Autodesk Inventor part; units mm, degrees
ref_plane "YZ Plane" through (0, 0, 0) normal (1, 0, 0) x (0, 1, 0)
ref_plane "XZ Plane" through (0, 0, 0) normal (0, 1, 0) x (-1, 0, 0)
ref_plane "XY Plane" through (0, 0, 0) normal (0, 0, 1) x (1, 0, 0)
ref_plane "Arbeitsebene1" through (-42.5, -18.05, -10) normal (0, -1, 0) x (1, 0, 0)
sketch "Skizze1" plane through (-42.5, -18.05, -10) normal (0, -1, 0) x (1, 0, 0)
  line L0 (45.91, 10.609) -> (59.4818, 10.609) construction
  line L1 (59.4818, 10.609) -> (63.5906, 10.303) construction
  line L2 (63.5906, 10.303) -> (66.1223, 6.4827) construction
  line L3 (66.1223, 6.4827) -> (69.15, 6.4827) construction
  spline S0 degree 4 poles (45.91, 10.609) (59.4818, 10.609) (63.5906, 10.303) (66.1223, 6.4827) (69.15, 6.4827) knots 1 1 1 1 1 2 2 2 2 2
  line L4 (46.0094, 12.5239) -> (59.5812, 12.5239) construction
  line L5 (59.5812, 12.5239) -> (63.69, 12.218) construction
  line L6 (63.69, 12.218) -> (66.2218, 8.3976) construction
  line L7 (66.2218, 8.3976) -> (69.15, 8.1737) construction
  spline S1 degree 4 poles (46.0094, 12.5239) (59.5812, 12.5239) (63.69, 12.218) (66.2218, 8.3976) (69.15, 8.1737) knots 1 1 1 1 1 2 2 2 2 2
  line L8 (46.0094, 12.5239) -> (45.91, 10.609)
  line L9 (69.15, 8.1737) -> (69.15, 6.4827)
  line L10 (42.5, 16.2648) -> (42.5, 4.43)
  point P0 (54.5567, 11.9133)
extrude "Extrusion1" add sketch "Skizze1" along normal mid plane 10
ref_plane "Arbeitsebene2" through (0, 0, 0) normal (0, 0, 1) x (1, 0, 0)
sketch "Skizze2" plane through (0, 0, 0) normal (0, 0, 1) x (1, 0, 0)
  line L0 (12.3, -18.05) -> (-2.05, -18.05)
  circle A0 centre (8.65, -14) radius 1.4
  circle A1 centre (8.65, -18.05) radius 1.6
  point P0 (0, 0)
  dimension "d2" = 3.2
extrude "Extrusion2" cut sketch "Skizze2" along normal mid plane 10 contours A1 L0 | L0 A1
mirror "Spiegeln1" about plane through (26.65, -18.05, -3.5173) normal (1, 0, 0) of "Extrusion1", "Extrusion2"
sketch "Skizze3" plane through (0, 0, 0) normal (0, 0, 1) x (1, 0, 0)
  line L0 (10.2456, -18.1688) -> (7.1543, -18.1688)
  line L1 (7.1543, -18.1688) -> (7.1543, 0.1733)
  line L2 (7.1543, 0.1733) -> (10.2456, 0.1733)
  line L3 (10.2456, 0.1733) -> (10.2456, -18.1688)
  point P0 (0, 0)
  point P1 (7.1543, -17.4817)
extrude "Extrusion3" cut sketch "Skizze3" along normal mid plane 10
fillet "Rundung1" radius 2 2 edges at (10.2456, -13.05, 1.4929) (7.1543, -13.05, 1.5517)
ref_plane "Arbeitsebene3" through (53.3, 0, 0) normal (0, 0, -1) x (-1, 0, 0)
properties part number "60_Planktoscope_Sampleholder_2"
Here's how the part is built. I have some questions about the finished solid (model axes, mm). A direction names the side the tool comes from. Round coordinates to 2 decimals unless told otherwise and drop trailing zeros. Use CSV: the item, a comma, the result in double quotes.
1) On a 3-axis mill with a long thin cutter (end or side, diameter ignored), from which of +Z, -Z, +X, -X, +Y, -Y can I reach the whole of each face in a straight line? I mean faces 4 (the cylindrical face through (6.55, -13.62, 1.54)), 5 (the cylindrical face through (45.92, -19.02, 1.51)). Say none if no direction works.
Taken from the geometry:
face 4,"+Z, -Z, +Y"
face 5,"+Z, -Z"
2) I'm going to push flat-ended pins straight in: P1, Ø3.5, axis at x = 44.65, y = -18.05, coming from the -Z side; P2, Ø1.5, axis at x = 11.5, y = -15.5, coming from the +Z side; P3, Ø2, axis at y = -15.5, z = 2, coming from the +X side. Where does each tip first touch, or does it pass through?
Taken from the geometry:
P1,"z = 0.53"
P2,"z = 2.44"
P3,"x = 49.87"
3) I want a section at A-A (z = 1). Count the separate pieces of the cut face and the enclosed holes in it, then the cut area to 3 significant figures.
Taken from the geometry:
separate pieces,"2"
enclosed holes,"1"
area,"309 mm^2"
4) If we mould it in two halves opening along Y, with no side actions, what happens to faces 1 (the flat face through (4, -13.05, 2)), 2 (the cylindrical face through (8.34, -19.62, 1.51)), 3 (the flat face through (49.84, -17.98, 1.55))? For each: pulls with the +Y half, pulls with the -Y half, needs draft (parallel to the pull), parting line crosses it, or undercut.
Taken from the geometry:
face 1,"pulls with the +Y half"
face 2,"undercut"
face 3,"needs draft"
5) I need wall thicknesses on line 1 along Y through (x, z) = (44.65, 1.7); line 2 along X through (y, z) = (-17.5, 0.75); line 3 along Z through (x, y) = (48, -14.75). Which ranges of each line are inside material? Lowest first, please. Write a range as [from, to].
Taken from the geometry:
line 1,"[-23.05, -19.65], [-16.45, -13.05]"
line 2,"[3.42, 7.15], [10.25, 20.97], [32.33, 43.15], [46.15, 49.88]"
line 3,"[0.61, 2.52]"
